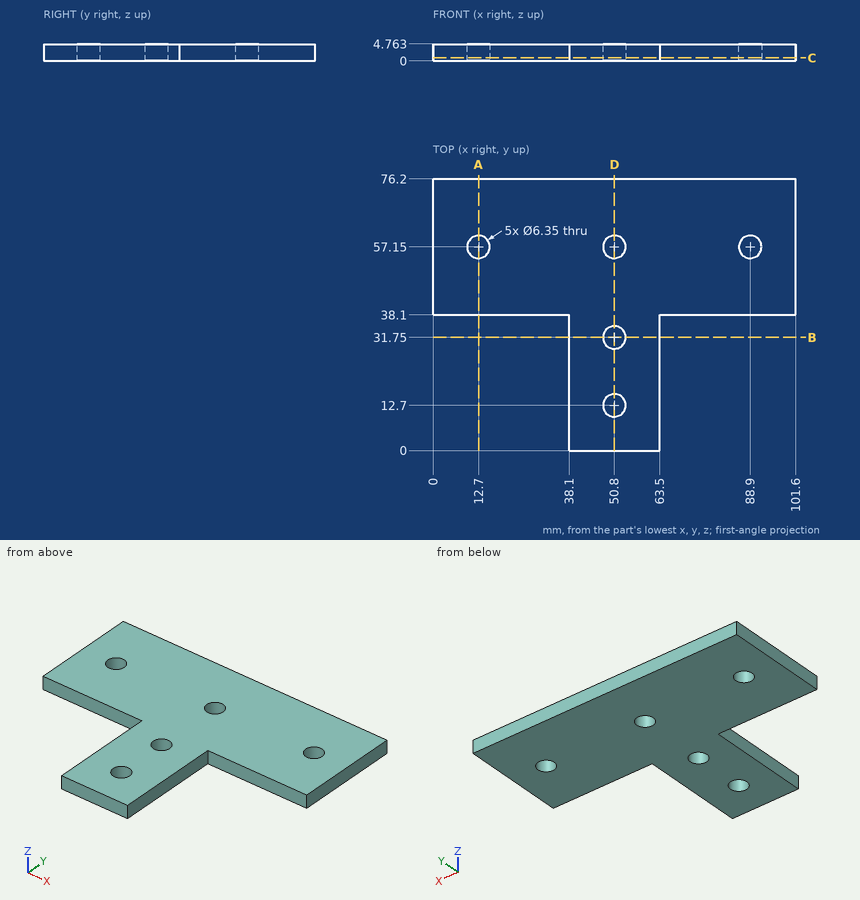
Study the drawing (mm; zero at the part's minimum x, y, z) and answer. Coordinates: 2 decimals unless noted, no trailing zeros. Write each loop counter-clockwise with the first axis right and the second up, starting at its lowest first coordinate (ties: lowest second). Pieces come first, ordered by that corner, then holes. Notation, with made-up numbers: (31, 81) - (48, 81) arc R8 cw to (48, 95) - close; hole circle Ø10 at (64.25, -26). An arc over 180 degrees is marked (long way). One line per question, with ' | ' between items.
1) Find section D-D, the plane x = 50.8. Determine the outline of the cut face in (y, z) (1 decimal), and give its area (3 significant figures).
Checks:
outline: (0, 0) - (9.5, 0) - (9.5, 4.8) - (0, 4.8) - close; (15.9, 0) - (28.6, 0) - (28.6, 4.8) - (15.9, 4.8) - close; (34.9, 0) - (54, 0) - (54, 4.8) - (34.9, 4.8) - close; (60.3, 0) - (76.2, 0) - (76.2, 4.8) - (60.3, 4.8) - close | area: 272 mm2
2) Flat-ended cylindrical pins translate along their axes: P1, Ø5, axis at x = 12.7, y = 57.15, coming from the -Z side; P2, Ø1, axis at y = 14.5, z = 3.5, coming from the +X side; P3, Ø2.5, axis at x = 88.5, z = 1.5, coming from the -Y side. Find the tip coordinate at first contact, or state that the pin passes through.
Checks:
P1: through | P2: x = 63.5 | P3: y = 38.1
3) Find section B-B, the plane y = 31.75. Determine the outline of the cut face in (x, z) (1 decimal).
Checks:
outline: (38.1, 0) - (47.6, 0) - (47.6, 4.8) - (38.1, 4.8) - close; (54, 0) - (63.5, 0) - (63.5, 4.8) - (54, 4.8) - close
4) Find section A-A, the plane x = 12.7. Determine the outline of the cut face in (y, z) (1 decimal).
Checks:
outline: (38.1, 0) - (54, 0) - (54, 4.8) - (38.1, 4.8) - close; (60.3, 0) - (76.2, 0) - (76.2, 4.8) - (60.3, 4.8) - close
5) Find section C-C, the plane z = 0.85. Give the number of separate pieces and of enclosed holes in the cut face, and give its area (3 significant figures).
Checks:
separate pieces: 1 | enclosed holes: 5 | area: 4,680 mm2
6) Consider probe 1 along Y at (x, z) = (50.8, 2.3) (1 decimal); probe 2 along Y at (x, z) = (88.9, 1.15) (1 decimal); probe 3 along X at (y, z) = (59, 3.8). Determine where each line is inside the solid, lowest interval first. Write a range as [from, to].
Checks:
probe 1: [0, 9.5], [15.9, 28.6], [34.9, 54], [60.3, 76.2] | probe 2: [38.1, 54], [60.3, 76.2] | probe 3: [0, 10.12], [15.28, 48.22], [53.38, 86.32], [91.48, 101.6]
